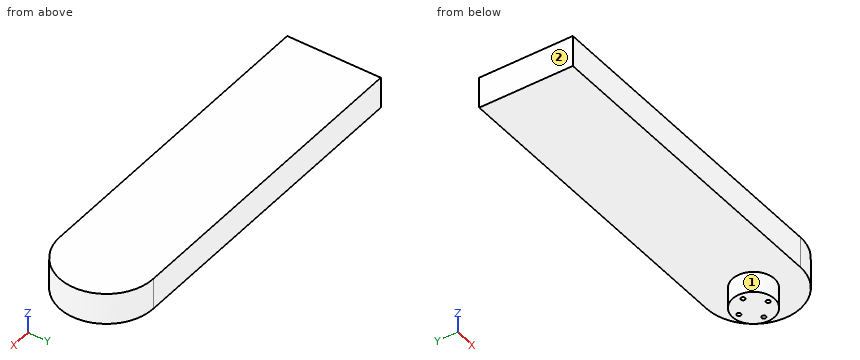
```python
from build123d import *

# Parameters (mm, degrees)
SKETCH_1_W          = 300
SKETCH_1_H          = 44.73
EXTRUDE_1_DEPTH     = 15
CUT_EXTRUDE_4_REACH = 305.687
SKETCH_6_R          = 10
EXTRUDE_2_DEPTH     = 10
SKETCH_7_R          = 1
CUT_EXTRUDE_6_DEPTH = 5


with BuildPart() as part:
    # 草图1 → 凸台-拉伸1 (new body)
    with BuildSketch(Plane.XY):
        with Locations((150, 22.365)):
            Rectangle(SKETCH_1_W, SKETCH_1_H)
    extrude(amount=EXTRUDE_1_DEPTH)

    # 草图4 → 切除-拉伸4 (cut, up to next)
    with BuildSketch(Plane.XY.offset(15), mode=Mode.PRIVATE) as cut_extrude_4_sk1:
        with BuildLine():
            Line((300, 44.73), (153.211623388, 44.73))
            ThreePointArc((153.211623388, 44.73), (175.576623388, 22.365), (153.211623388, 0))
            Line((153.211623388, 0), (300, 0))
            Line((300, 0), (300, 44.73))
        make_face()
    cut_extrude_4_tool1 = extrude(cut_extrude_4_sk1.sketch, amount=-CUT_EXTRUDE_4_REACH, mode=Mode.PRIVATE) & part.part
    add(cut_extrude_4_tool1.solids().sort_by_distance((235.292113, 22.365, 15))[0], mode=Mode.SUBTRACT)

    # 草图6 → 凸台-拉伸2 (add)
    with BuildSketch(Plane(origin=(0, 0, 0), x_dir=(-1, 0, 0), z_dir=(0, 0, -1))):
        with Locations((-153.211623388, 22.365)):
            Circle(SKETCH_6_R)
    extrude(amount=EXTRUDE_2_DEPTH)

    # 草图7 → 切除-拉伸6 (cut)
    with BuildSketch(Plane(origin=(0, 0, -10), x_dir=(-1, 0, 0), z_dir=(0, 0, -1))):
        with Locations((-153.211623388, 29.365)):
            Circle(SKETCH_7_R)
        with Locations((-146.211623388, 22.365)):
            Circle(SKETCH_7_R)
        with Locations((-153.211623388, 15.365)):
            Circle(SKETCH_7_R)
        with Locations((-160.211623388, 22.365)):
            Circle(SKETCH_7_R)
    extrude(amount=-CUT_EXTRUDE_6_DEPTH, mode=Mode.SUBTRACT)


solid = part.part
```
Build history of the part. All positions in model axes, mm. Face numbers are marked on the shaded views. A direction names the side the tool comes from. Round coordinates to 2 decimals unless told otherwise and drop trailing zeros. Order: outer loops, then holes, each group sorted by start corner. A loop starts at its lowest first (then second) coordinate and runs counter-clockwise, first axis right, second up. Notation, with made-up numbers: (51, -9.75) - (62, -9.75) arc R6 cw to (62, -4.75) - close; hole circle Ø2 at (16.25, -21.5). An arc over 180 degrees is marked (long way). Use a Markdown table: item, result.
1) Flat gauge pins, fed straight in: pin 1 Ø8 at (y, z) = (32.5, -3.5) entering from -X; pin 2 Ø0.6 at (x, y) = (153, 29) entering from -Z; pin 3 Ø22.5 at (x, y) = (116, 29) entering from -Z. Where does each tip first touch, or does it go through?
Recorded:
| item | result |
|---|---|
| pin 1 | stops at x = 0 |
| pin 2 | stops at z = -5 |
| pin 3 | stops at z = 0 |
2) Saw through at C-C on x = 140. Write the cut outline in (y, z), and give its area (3 significant figures).
Recorded:
| item | result |
|---|---|
| outline | (0, 0) - (44.73, 0) - (44.73, 15) - (0, 15) - close |
| area | 671 mm² |
3) Saw through at D-D on z = -2.5. Write the cut outline in (x, y) (3 decimals), and give its area (3 significant figures).
Recorded:
| item | result |
|---|---|
| outline | circle Ø20 at (153.212, 22.365) |
| area | 314 mm² |
4) Saw through at B-B on y = 18. Write the cut outline in (x, z), and give its area (3 significant figures).
Recorded:
| item | result |
|---|---|
| outline | (0, 0) - (144.21, 0) - (144.21, -10) - (162.21, -10) - (162.21, 0) - (175.15, 0) - (175.15, 15) - (0, 15) - close |
| area | 2,810 mm² |
5) Tool access for the marked faces 1 and 2: list every direction of +Z, -Z, +X, -X, +Y, -Y with a clear straight run to the whole face (end or side of a thin tool).
Recorded:
| item | result |
|---|---|
| face 1 | -Z |
| face 2 | +Z, -Z, -X, +Y, -Y |
6) Saw through at A-A on z = 11.75. Write the cut outline in (x, y) (3 decimals), and give its area (3 significant figures).
Recorded:
| item | result |
|---|---|
| outline | (0, 0) - (153.212, 0) arc R22.365 ccw to (153.212, 44.73) - (0, 44.73) - close |
| area | 7,640 mm² |
7) Wall check: L1, parallel to X at y = 22, z = -2.25; L2, parallel to Z at x = 87, y = 4.5; L3, parallel to X at y = 25, z = 8.5. Give the ranges that are in metal, low to high.
Recorded:
| item | result |
|---|---|
| L1 | x = 143.22 to 163.2 |
| L2 | z = 0 to 15 |
| L3 | x = 0 to 175.42 |
